Part model, mm, in its own coordinate system. A direction names the side the tool comes from. Give positions to 0.01 mm unless a question says otherwise; leave off trailing zeros. Order: outer loops, then holes, each group sorted by start corner. A loop starts at its lowest first (then second) coordinate and runs counter-clockwise, first axis right, second up. Notation, with made-up numbers: M 82,26 L 100,26 A19 ccw 100,63 Z; hole C 12,1.5 d11. An arc over 180 degrees is marked long. Answer as a JSON object with one key per item and string values.
from build123d import *

# Parameters (mm, degrees)
F0_R     = 6
F1_DEPTH = 25
F3_DEPTH = 12.5
F4_R     = 5


with BuildPart() as f1:
    # F0 (on Front) → F1 (new body)
    with BuildSketch(Plane.XZ):
        with BuildLine():
            ThreePointArc((9.604686, -8), (11.753905, -4.253905), (12.5, 0))
            ThreePointArc((12.5, 0), (11.753905, 4.253905), (9.604686, 8))
            ThreePointArc((9.604686, 8), (-12.5, 0), (9.604686, -8))
        make_face()
        Circle(F0_R, mode=Mode.SUBTRACT)
        with BuildLine():
            ThreePointArc((9.604686, 8), (11.753905, 4.253905), (12.5, 0))
            ThreePointArc((12.5, 0), (11.753905, -4.253905), (9.604686, -8))
            Line((9.604686, -8), (79, -8))
            ThreePointArc((79, -8), (75, 0), (79, 8))
            Line((79, 8), (9.604686, 8))
        make_face()
        with BuildLine():
            ThreePointArc((95, 0), (89.472136, 8.944272), (79, 8))
            ThreePointArc((79, 8), (75, 0), (79, -8))
            ThreePointArc((79, -8), (89.472136, -8.944272), (95, 0))
        make_face()
        with Locations((85, 0)):
            Circle(F0_R, mode=Mode.SUBTRACT)
    extrude(amount=F1_DEPTH)

    # F2 (on Top) → F3 (intersect, symmetric)
    with BuildSketch(Plane.XY):
        Polygon((20, 0), (-12.5, 0), (-12.5, -8), (19.300091, -8), (70.341627, -17), (95, -17), (95, -9), (71.041536, -9), align=None)
    extrude(amount=F3_DEPTH, both=True, mode=Mode.INTERSECT)

    # F4
    f4_edges = [f1.edges().sort_by_distance(p)[0] for p in [
        (79, -13, 8),
        (9.604686, -4, 8),
        (79, -13, -8),
        (9.604686, -4, -8),
    ]]
    fillet(f4_edges, radius=F4_R)


solid = f1.part
1. Pin check, flat tips, straight feed: P1, Ø7, axis at x = 85, z = 0, coming from the -Y side; P2, Ø5, axis at x = 33.5, y = -8.5, coming from the +Z side; P3, Ø5, axis at x = 81, y = -11.5, coming from the -Z side; P4, Ø1, axis at y = -9, z = -9.5, coming from the +X side. Stop position of each tip, or through.
Worked answers:
{"P1": "passes through", "P2": "stops at z = 8", "P3": "stops at z = -9.89", "P4": "stops at x = 89.36"}
2. Cut at B-B on x = 85. Give the cut face in (y, z), plus the area to 3 significant figures.
Worked answers:
{"outline": "M -17,-10 L -9,-10 L -9,-6 L -17,-6 Z; M -17,6 L -9,6 L -9,10 L -17,10 Z", "area": "64.0 mm^2"}
3. Probe line 1 along Z through (x, y) = (0, -3.25); line 2 along Y through (x, z) = (-3.5, -6.25); line 3 along Z through (x, y) = (20.5, -5.25). List the from-to ranges inside material, lowest first.
Worked answers:
{"line 1": "z = -12.5 to -6, 6 to 12.5", "line 2": "y = -8 to 0", "line 3": "z = -8 to 8"}
4. Which spindle directions (+Z, -Z, +X, -X, +Y, -Y) get a long thin tool onto all of the face, cutting with end or side? Do faces 1 (the flat face through (7, -8, 0)), 2 (the flat face through (78, -9, 0)), 3 (the flat face through (44, -8, -8)). Say none if no direction does.
Worked answers:
{"face 1": "+Z, -Z, -X, -Y", "face 2": "+Z, -Z, +X, +Y", "face 3": "-Z, +Y, -Y"}
5. Cut at A-A on x = 0. Give the cut face in (y, z).
Worked answers:
{"outline": "M -8,-12.5 L 0,-12.5 L 0,-6 L -8,-6 Z; M -8,6 L 0,6 L 0,12.5 L -8,12.5 Z"}
6. Cut at D-D on z = 3.5. Give the cut face in (x, y).
Worked answers:
{"outline": "M -12,-8 L -4.87,-8 L -4.87,0 L -12,0 Z; M 4.87,-8 L 19.3,-8 L 70.34,-17 L 80.13,-17 L 80.13,-9 L 71.04,-9 L 20,0 L 4.87,0 Z; M 89.87,-17 L 94.37,-17 L 94.37,-9 L 89.87,-9 Z"}
7. Two-plate mould, pull along X, no slides. Class faces 4 (the cylindrical face through (78.79, -13.056, -8.165)), 5 (the flat face through (77, -17, 0)), 6 (the cylindrical face through (-6, -4, 0)): +X half, -X half, draft (parallel to the pull), parting line (faces both ways), or undercut.
Worked answers:
{"face 4": "-X half", "face 5": "draft", "face 6": "undercut"}
8. Cut at C-C on y = -11.75. Give the cut face in (x, z), plus the area to 3 significant figures.
Worked answers:
{"outline": "M 40.57,-8 L 77.52,-8 A5 cw 80.01,-8.67 A10 ccw long 80.01,8.67 A5 cw 77.52,8 L 40.57,8 Z; hole C 85,0 d12", "area": "772 mm^2"}
